Input: dimensioned drawing with shaded views. Units: mm. Origin: part minimum x, y, z. A direction names the side the tool comes from. Give positions to 0.01 mm unless a question says otherwise; leave off trailing zeros. Order: outer loops, then holes, each group sorted by start corner. A loop starts at its lowest first (then second) coordinate and runs counter-clockwise, first axis right, second up.
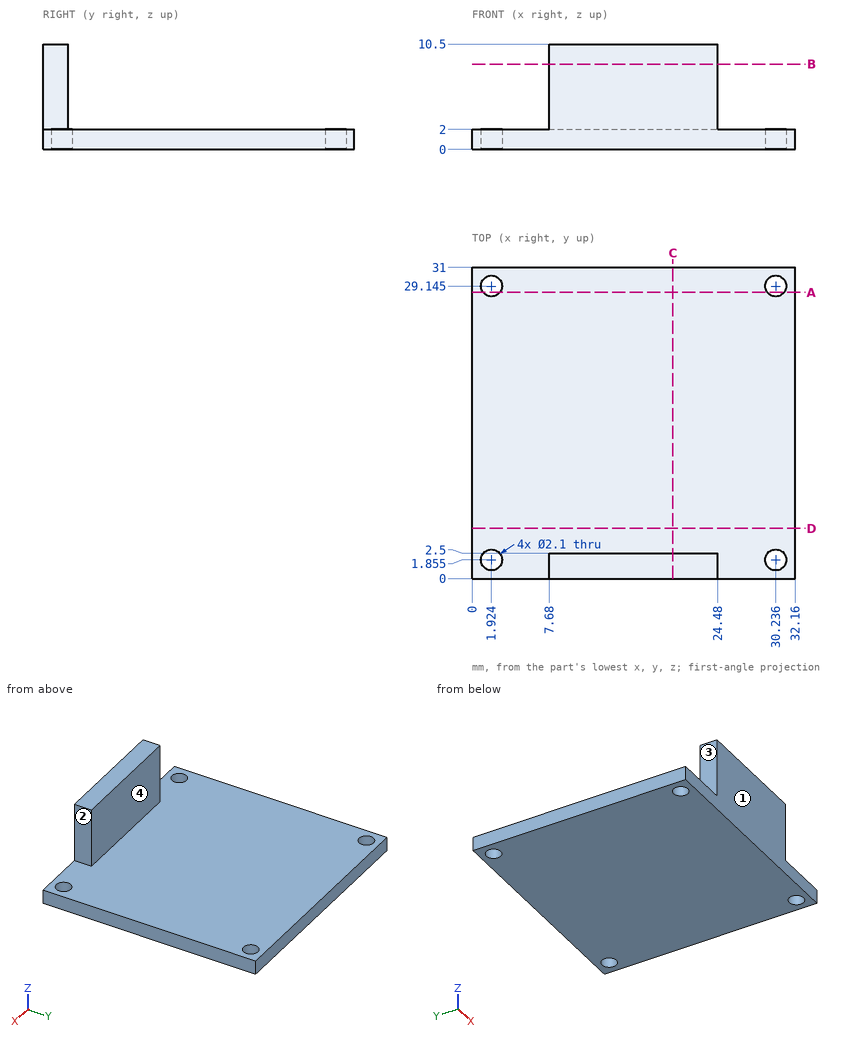
1) Section query B-B, the plane z = 8.5. Return the cut outline in (x, y), and give its area (3 significant figures).
Report:
outline: (7.68, 0) - (24.48, 0) - (24.48, 2.5) - (7.68, 2.5) - close
area: 42.0 mm2
2) Section query A-A, the plane y = 28.5. Return the cut outline in (x, z).
Report:
outline: (0, 0) - (1.1, 0) - (1.1, 2) - (0, 2) - close; (2.75, 0) - (29.41, 0) - (29.41, 2) - (2.75, 2) - close; (31.06, 0) - (32.16, 0) - (32.16, 2) - (31.06, 2) - close
3) Pin query (flat end, axial travel): pin 1 (6 mm diameter, centred on x = 15, y = 18, fed in from +Z); pin 2 (3 mm diameter, centred on x = 20.5, z = 5.5, fed in from +Y); pin 3 (2 mm diameter, centred on y = 0.5, z = 5, fed in from -X). Return the tip coordinate at first contact, or that it passes through.
Report:
pin 1: stops at z = 2
pin 2: stops at y = 2.5
pin 3: stops at x = 7.68
4) Material intervals for L1, parallel to Z at x = 12, y = 9; L2, parallel to Y at x = 21.5, z = 7.25; L3, parallel to X at y = 1.5, z = 7.5, sorted ascending.
Report:
L1: z = 0 to 2
L2: y = 0 to 2.5
L3: x = 7.68 to 24.48
5) Section query D-D, the plane y = 5. Return the cut outline in (x, z).
Report:
outline: (0, 0) - (32.16, 0) - (32.16, 2) - (0, 2) - close
6) Section query C-C, the plane x = 20. Return the cut outline in (y, z).
Report:
outline: (0, 0) - (31, 0) - (31, 2) - (2.5, 2) - (2.5, 10.5) - (0, 10.5) - close
7) Reachability of the marked faces 1, 2, 3 and 4 from +Z, -Z, +X, -X, +Y, -Y: full face, straight path, thin tool, end or side. Return the list, or none.
Report:
face 1: +Z, -Z, +X, -X, -Y
face 2: +Z, +X, +Y, -Y
face 3: +Z, -X, +Y, -Y
face 4: +Z, +X, -X, +Y
